```python
from build123d import *

# Parameters (mm, degrees)
PAD011_DEPTH    = 1.7
SKETCH021_R     = 2.475826
SKETCH021_R_2   = 2.481394
SKETCH021_R_3   = 2.464202
SKETCH021_R_4   = 2.48
POCKET021_DEPTH = 2
SKETCH022_W     = 1.6
SKETCH022_H     = 2.6
PAD012_DEPTH    = 1.1
SKETCH025_W     = 3.5
SKETCH025_H     = 6
PAD014_DEPTH    = 2.5
PAD015_DEPTH    = 2


with BuildPart() as part:
    # MirroredSketch016 → Pad011 (new body)
    with BuildSketch(Plane.XY):
        Polygon((18.615471, 0), (55.795471, 0), (66.524073, -14.707193), (104.028226, -19.584789), (119.695382, -28.648464), (133.795471, -4.157341), (133.795471, 56.252659), (113.045471, 56.252659), (113.045471, 58.502659), (94.055471, 58.502659), (94.055471, 61.002659), (75.055471, 61.002659), (75.055471, 63.252659), (57.055471, 63.252659), (57.055471, 61.002659), (38.045471, 61.002659), (38.045471, 56.25), (18.615471, 56.25), align=None)
    extrude(amount=PAD011_DEPTH)

    # Sketch021 → Pocket021 (cut)
    with BuildSketch(Plane.XY):
        with Locations((61.841369, 1.48161)):
            Circle(SKETCH021_R)
        with Locations((108.248942, -6.275442)):
            Circle(SKETCH021_R_2)
        with Locations((94.502421, 41.204275)):
            Circle(SKETCH021_R_3)
        with Locations((37.563327, 37.48)):
            Circle(SKETCH021_R_4)
        with Locations((37.51863, 18.740053)):
            Circle(SKETCH021_R_4)
    extrude(amount=POCKET021_DEPTH, mode=Mode.SUBTRACT)

    # Sketch022 → Pad012 (join)
    with BuildSketch(Plane.XY.offset(-1.1)):
        with Locations((48.005105, 34.081744)):
            Rectangle(SKETCH022_W, SKETCH022_H)
    extrude(amount=PAD012_DEPTH)

    # Sketch025 → Pad014 (join)
    with BuildSketch(Plane(origin=(-22, 35, 1.7), x_dir=(1, 0, 0), z_dir=(0, 0, 1))):
        with Locations((137.295471, -18.767341)):
            Rectangle(SKETCH025_W, SKETCH025_H)
    extrude(amount=PAD014_DEPTH)

    # Sketch026 → Pad015 (join)
    with BuildSketch(Plane.XY.offset(1.7)):
        Polygon((132.98, 3.032659), (130.18, 3.032659), (130.18, 9.832659), (132.98, 9.832659), (132.98, 7.932659), (134.48, 7.932659), (134.48, 6.532659), (132.98, 6.532659), align=None)
    extrude(amount=PAD015_DEPTH)


with BuildPart() as part_1:
    # Body009 placement: moved
    add(part.part.moved(Location((0, 0, 3.3))))


solid = part_1.part
```
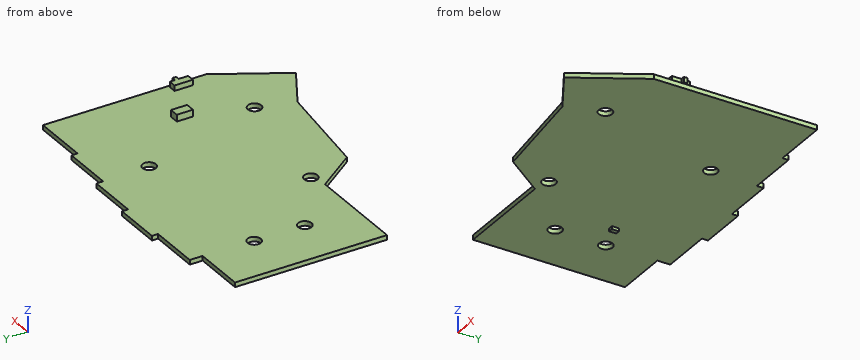
Read the model definition and answer for the solid it produces. Units are mm, in the model's axes. Round coordinates to 2 decimals unless told otherwise and drop trailing zeros. Write each loop counter-clockwise with the first axis right and the second up, starting at its lowest first coordinate (ties: lowest second). Pieces come first, ordered by that corner, then holes. Notation, with made-up numbers: (77, 82.5) - (108, 82.5) arc R31 ccw to (108, 112.5) - close; hole circle Ø10 at (9.5, 34.5). An arc over 180 degrees is marked (long way). One line per item, written item: value.
Q1. Straight lines are drawn through the part: line 1 (X direction, y = 37.48, z = 3.7); line 2 (Z direction, x = 122, y = 16); line 3 (X direction, y = 56.5, z = 4.85). For each, find the intervals that lie inside material, in ascending order. Write a range as from..to.
The answers:
line 1: x = 18.62..35.08, 40.04..133.8
line 2: z = 3.3..5
line 3: x = 38.05..113.05
Q2. Each of these flat-tipped pins is pushed along its axis until it touches: P1, Ø5, axis at x = 76, y = -2, coming from the +Z side; P2, Ø1.9, axis at y = 60, z = 4.5, coming from the +X side; P3, Ø1.2, axis at y = 34, z = 2.5, coming from the -X side; P4, Ø4, axis at x = 37.52, y = 18.74, coming from the -Z side. Where does it stop, or does it pass through?
The answers:
P1: stops at z = 5
P2: stops at x = 94.06
P3: stops at x = 47.21
P4: passes through
Q3. Find section B-B (z = 4.15). Determine the outline of the cut face in (x, y), and give its area (3 significant figures).
The answers:
outline: (18.62, 0) - (55.8, 0) - (66.52, -14.71) - (104.03, -19.58) - (119.7, -28.65) - (133.8, -4.16) - (133.8, 56.25) - (113.05, 56.25) - (113.05, 58.5) - (94.06, 58.5) - (94.06, 61) - (75.06, 61) - (75.06, 63.25) - (57.06, 63.25) - (57.06, 61) - (38.05, 61) - (38.05, 56.25) - (18.62, 56.25) - close; hole circle Ø4.96 at (37.52, 18.74); hole circle Ø4.96 at (37.56, 37.48); hole circle Ø4.95 at (61.84, 1.48); hole circle Ø4.93 at (94.5, 41.2); hole circle Ø4.96 at (108.25, -6.28)
area: 8,060 mm2
Q4. Find section A-A (y = 37.48). Determine the outline of the cut face in (x, z).
The answers:
outline: (18.62, 3.3) - (35.08, 3.3) - (35.08, 5) - (18.62, 5) - close; (40.04, 3.3) - (133.8, 3.3) - (133.8, 5) - (40.04, 5) - close
Q5. Find section C-C (y = 47). Determine the outline of the cut face in (x, z).
The answers:
outline: (18.62, 3.3) - (133.8, 3.3) - (133.8, 5) - (18.62, 5) - close
Q6. Find section D-D (x = 79). Determine the outline of the cut face in (y, z), and give its area (3 significant figures).
The answers:
outline: (-16.33, 3.3) - (61, 3.3) - (61, 5) - (-16.33, 5) - close
area: 131 mm2
